The listing builds one solid part. Answer for the finished solid, in the listing's coordinates (mm). A direction names the side the tool comes from. Coordinates: 2 decimals unless noted, no trailing zeros. Order: outer loops, then holes, each group sorted by start corner. A loop starts at its lowest first (then second) coordinate and runs counter-clockwise, first axis right, second up. Notation, with made-up numbers: (41.5, 27) -> (58.5, 27) arc R8 ccw to (58.5, 41) -> close; hole circle Ø10 at (65, 51.5). An arc over 180 degrees is marked (long way). Write item = value, one per line.
from build123d import *

# Parameters (mm, degrees)
SKETCH1_R                = 5
SKETCH1_R_2              = 3.95
BOSS_EXTRUDE1_DEPTH      = 8
BOSS_EXTRUDE2_DEPTH      = 5
BOSS_EXTRUDE2_DEPTH_BACK = 5
CUT_EXTRUDE1_DEPTH       = 18.492855685
CUT_EXTRUDE1_DEPTH_BACK  = 18.492855685
SKETCH4_R                = 1.3


with BuildPart() as part:
    # Sketch1 → Boss-Extrude1 (new body)
    with BuildSketch(Plane.XY):
        Circle(SKETCH1_R)
        Circle(SKETCH1_R_2, mode=Mode.SUBTRACT)
    extrude(amount=BOSS_EXTRUDE1_DEPTH)

    # Sketch3 → Boss-Extrude2 (add, two sides: drawn at the far end of the back side and taken through both)
    with BuildSketch(Plane(origin=(0, 0, 0), x_dir=(1, 0, 0), z_dir=(0, 1, 0)).offset(-BOSS_EXTRUDE2_DEPTH_BACK)):
        Polygon((5, -16), (-5, -8), (5, -8), align=None)
    extrude(amount=BOSS_EXTRUDE2_DEPTH + BOSS_EXTRUDE2_DEPTH_BACK)

    # Sketch4 → Cut-Extrude1 (cut, two sides: drawn at the far end of the back side and taken through both)
    with BuildSketch(Plane(origin=(0, 0, 0), x_dir=(1, 0, 0), z_dir=(0, 1, 0)).offset(-CUT_EXTRUDE1_DEPTH_BACK)):
        with Locations(Location((0, -3, 0), (0, 0, 270))):
            Circle(SKETCH4_R)
    extrude(amount=CUT_EXTRUDE1_DEPTH + CUT_EXTRUDE1_DEPTH_BACK, mode=Mode.SUBTRACT)


solid = part.part
Q1. Section A-A, the plane z = 3 is taken. Give the vertices of the cut face in (x, y), plus the area to 3 significant figures.
The answers:
outline = (-1.3, -4.83) -> (-1.3, -3.73) arc R3.95 cw to (-1.3, 3.73) -> (-1.3, 4.83) arc R5 ccw to start; (1.3, -4.83) arc R5 ccw to (1.3, 4.83) -> (1.3, 3.73) arc R3.95 cw to (1.3, -3.73) -> close
area = 24.0 mm2
Q2. A tool of negligible diameter and unlimited length cuts with its end or side. For faces 1 (the face through (0, 0, 8)), 2 (the face through (4, -4, 8)), 3 (the face through (-4, 4, 8)), 4 (the face through (4, 4, 8)), from which of +Z, -Z, +X, -X, +Y, -Y can it reach the whole face along a straight path? Write none if from no direction.
The answers:
face_1 = -Z
face_2 = -Z, +X, -Y
face_3 = -Z, -X, +Y
face_4 = -Z, +X, +Y
Q3. Section C-C, the plane x = -2 is taken. Give the vertices of the cut face in (y, z), plus the area to 3 significant figures.
The answers:
outline = (-5, 8) -> (-4.58, 8) -> (-4.58, 0) -> (-3.41, 0) -> (-3.41, 8) -> (3.41, 8) -> (3.41, 0) -> (4.58, 0) -> (4.58, 8) -> (5, 8) -> (5, 10.4) -> (-5, 10.4) -> close
area = 42.8 mm2
Q4. Section B-B, the plane x = -0.75 is taken. Give the vertices of the cut face in (y, z).
The answers:
outline = (-5, 8) -> (-4.94, 8) -> (-4.94, 4.06) -> (-3.88, 4.06) -> (-3.88, 8) -> (3.88, 8) -> (3.88, 4.06) -> (4.94, 4.06) -> (4.94, 8) -> (5, 8) -> (5, 11.4) -> (-5, 11.4) -> close; (-4.94, 0) -> (-3.88, 0) -> (-3.88, 1.94) -> (-4.94, 1.94) -> close; (3.88, 0) -> (4.94, 0) -> (4.94, 1.94) -> (3.88, 1.94) -> close
Q5. Section D-D, the plane y = 2 is taken. Give the vertices of the cut face in (x, z).
The answers:
outline = (-5, 8) -> (-4.58, 8) -> (-4.58, 0) -> (-3.41, 0) -> (-3.41, 8) -> (3.41, 8) -> (3.41, 0) -> (4.58, 0) -> (4.58, 8) -> (5, 8) -> (5, 16) -> close
Q6. This flat-tipped pin is pushed along its axis until it touches: pin 1 Ø1 at (x, y) = (-1.5, 0) entering from -Z. Where does it stop, or does it pass through?
The answers:
pin_1 = 8
Q7. The mould has two halves that part along Y. Classify faces 5 (the face through (2.307, -4.436, 3.944)), 6 (the face through (-4, -4, 8)), 7 (the face through (3.768, 1.186, 3.944)): released by +Y, released by -Y, zero draft, split by the parting line, or undercut.
The answers:
face_5 = split by the parting line
face_6 = zero draft
face_7 = undercut
Q8. Find the intervals of material crossed by line 1 along Y through (x, z) = (0, 5.5); line 2 along Z through (x, y) = (0, -4.3); line 3 along X through (y, z) = (4.55, 3), in increasing order.
The answers:
line_1 = -5 to -3.95, 3.95 to 5
line_2 = 0 to 1.7, 4.3 to 12
line_3 = -2.07 to -1.3, 1.3 to 2.07
